```python
from build123d import *

# Parameters (mm, degrees)
SKETCH1_R           = 1.5
BOSS_EXTRUDE1_DEPTH = 5
FILLET2_R           = 0.4
CHAMFER1_SIZE       = 0.4


with BuildPart() as part:
    # Sketch1 → Boss-Extrude1 (new body)
    with BuildSketch(Plane(origin=(0, 0, 0), x_dir=(1, 0, 0), z_dir=(0, 1, 0))):
        with Locations(Location((0, 0, 0), (0, 0, 270))):
            Circle(SKETCH1_R)
    extrude(amount=BOSS_EXTRUDE1_DEPTH)

    # Sketch3 → Revolve1 (revolve)
    with BuildSketch(Plane.XY):
        with BuildLine():
            Line((0, 5), (-3, 5))
            ThreePointArc((-3, 5), (-1.802775638, 6.454163457), (0, 7))
            Line((0, 7), (0, 5))
        make_face()
    revolve(axis=Axis((0, 7, 0), (0, -1, 0)))

    # Fillet2
    fillet2_edges = [part.edges().sort_by_distance(p)[0] for p in [
        (0, 5, -1.5),
    ]]
    fillet(fillet2_edges, radius=FILLET2_R)

    # Chamfer1
    # the kernel refuses this chamfer: 0.4, 0.305882353 mm, written as the material it takes off along each edge
    with BuildSketch(Plane(origin=(0, 5, 0), x_dir=(-1, 0, 0), z_dir=(0, 0, 1))) as chamfer1_piece_1:
        with BuildLine():
            Line((3 - CHAMFER1_SIZE, 0), (2.871730525, -0.271730525))
            ThreePointArc((2.871730525, -0.271730525), (2.93785488, -0.139787287), (3, 0))
            Line((3, 0), (3 - CHAMFER1_SIZE, 0))
        make_face()
    revolve(axis=Axis((0, 5, 0), (0, -1, 0)), mode=Mode.SUBTRACT)


solid = part.part
```
Geometry check sheet. Reference: the model listing, model coordinates, mm. A direction names the side the tool comes from. Give positions to 0.01 mm unless a question says otherwise; leave off trailing zeros. Write each loop counter-clockwise with the first axis right and the second up, starting at its lowest first coordinate (ties: lowest second). Pieces come first, ordered by that corner, then holes.
1) Section check D-D, the plane y = 3.75. Record the boundary of the cut face in (x, z).
2) Gauge pin test, flat ends, axial feed: pin 1 (1.6 mm diameter, centred on x = 0.5, z = 0, fed in from -Y); pin 2 (2 mm diameter, centred on y = 1.5, z = -0.5, fed in from -X). Record the tip position at first contact, or that the pin passes through.
3) Section check C-C, the plane y = 6.75. Record the boundary of the cut face in (x, z).
4) Access from +Z, -Z, +X, -X, +Y, -Y to the whole of each face (thin tool, end or side, straight path). Record for faces 1 (the flat face through (1, 5, 2)), 2 (the flat face through (0, 0, 0)).
5) Section check A-A, the plane z = 0. Record the boundary of the cut face in (x, y).
6) Material ranges on L1, parallel to X at y = 4.5, z = 0.7; L2, parallel to Y at x = -0.55, z = -0.8; L3, parallel to Z at x = 0.75, y = 2, recorded low to high.
7) Section check B-B, the plane x = 0. Record the boundary of the cut face in (y, z), and give its area (3 significant figures).
Computed:
1. outline: circle Ø3 at (0, 0)
2. pin 1: stops at y = 0
2. pin 2: stops at x = -1.5
3. outline: circle Ø2.5 at (0, 0)
4. face 1: -Y
4. face 2: +Z, -Z, +X, -X, -Y
5. outline: (-2.87, 5.27) - (-2.6, 5) - (-1.9, 5) arc R0.4 cw to (-1.5, 4.6) - (-1.5, 0) - (1.5, 0) - (1.5, 4.6) arc R0.4 cw to (1.9, 5) - (2.6, 5) - (2.87, 5.27) arc R3.25 ccw to start
6. L1: x = -1.33 to 1.33
6. L2: y = 0 to 6.85
6. L3: z = -1.3 to 1.3
7. outline: (0, -1.5) - (4.6, -1.5) arc R0.4 cw to (5, -1.9) - (5, -2.6) - (5.27, -2.87) arc R3.25 ccw to (5.27, 2.87) - (5, 2.6) - (5, 1.9) arc R0.4 cw to (4.6, 1.5) - (0, 1.5) - close
7. area: 23.6 mm2
